Source: CAD feature listing. Evaluate the final solid. Frame: model axes, mm. Face numbers are marked on the shaded views. A direction names the side the tool comes from. Give positions to 0.01 mm unless a question says otherwise; leave off trailing zeros. Order: outer loops, then holes, each group sorted by start corner. A loop starts at its lowest first (then second) coordinate and runs counter-clockwise, first axis right, second up. Notation, with made-up numbers: (31, -13) - (36, -13) arc R15 cw to (36, 15) - close; hole circle Ø6 at (-2.5, 67.25). An arc over 180 degrees is marked (long way). Use CSV: the item, a comma, the result in double quotes.
```python
from build123d import *

# Parameters (mm, degrees)
F1_DEPTH = 49.022
F2_T     = -2.54
F4_W     = 49.022
F4_H     = 1.7985738814
F5_DEPTH = 9.652


with BuildPart() as f1:
    # F0 (on Right) → F1 (new body)
    with BuildSketch(Plane.YZ):
        Polygon((1.5098481488, -2.5384752646), (-15.0794390421, -5.5547094899), (-14.0161000537, -11.4030735567), (1.5098481488, -11.4030735567), (2.9737947043, -19.4547791034), (2.9737947043, -46.7351712286), (-5.6977379136, -46.7351712286), (-5.6886866642, -48.53374511), (16.9632527977, -48.6290739331), (16.9632527977, 26.2930374593), (11.1203547567, 26.2930374593), align=None)
    extrude(amount=-F1_DEPTH)

    # F2
    f2_openings = [f1.faces().sort_by_distance(p)[0] for p in [
        (-24.511, 6.315101, 11.877281),
        (-24.511, -6.784795, -4.046592),
    ]]
    offset(amount=F2_T, openings=f2_openings, kind=Kind.INTERSECTION)

    # F4 (on face) → F5 (join)
    with BuildSketch(Plane.XZ.offset(-2.9737947043)):
        with Locations((-24.511, -47.6344581693)):
            Rectangle(F4_W, F4_H)
    extrude(amount=F5_DEPTH)


with BuildPart() as f8_1:
    # F8: copy of F1
    add(f1.part)


solid = f1.part
```
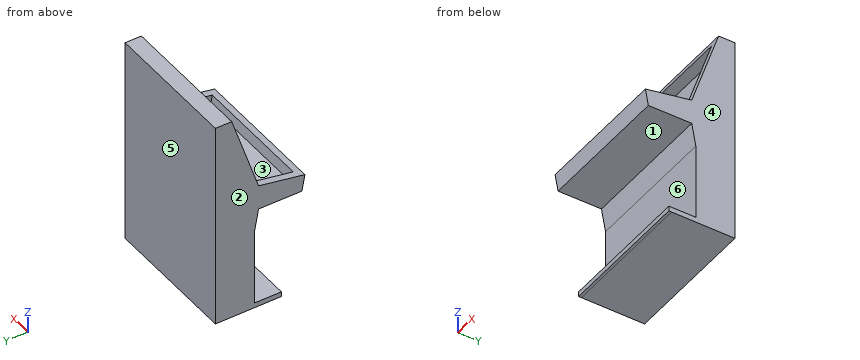
Item 1: Section C-C on y = 8. Return the cut outline in (x, z).
Filled in:
outline,"(-49.02, -48.59) - (0, -48.59) - (0, 16.93) - (-2.54, 16.93) - (-2.54, -46.05) - (-46.48, -46.05) - (-46.48, 16.93) - (-49.02, 16.93) - close"
Item 2: Mould query, pull axis X, two halves, no side actions, for the marked faces 1, 2, 3 and 4. Classes: released by +X, released by -X, zero draft, split by the parting line, or undercut.
Filled in:
face 1,"zero draft"
face 2,"released by -X"
face 3,"undercut"
face 4,"released by +X"
Item 3: Section B-B on x = -39.5. Return the cut outline in (y, z), then the cut area to 3 significant figures.
Filled in:
outline,"(-15.08, -5.55) - (-14.02, -11.4) - (1.51, -11.4) - (2.97, -19.45) - (2.97, -46.74) - (-6.68, -46.74) - (-6.68, -48.53) - (-5.69, -48.53) - (16.96, -48.63) - (16.96, 26.29) - (11.12, 26.29) - (10.27, 23.75) - (14.42, 23.75) - (14.42, -46.08) - (5.51, -46.04) - (5.51, -19.23) - (3.63, -8.86) - (-11.9, -8.86) - (-12.58, -5.1) - close"
area,"390 mm2"
Item 4: Set-up query: the marked faces 5 and 6. Return all of +Z, -Z, +X, -X, +Y, -Y with unobstructed straight access to the full face (end or side cutting, diameter ignored); none if empty.
Filled in:
face 5,"+Z, -Z, +X, -X, +Y"
face 6,"+X, -X, -Y"
Item 5: First-contact query: pin 1 (12 mm diameter, centred on x = -30.5, y = 0, fed in from +Z); pin 2 (0.5 mm diameter, centred on x = -33, y = -6.5, fed in from -Z); pin 3 (22 mm diameter, centred on x = -23.5, z = -32.5, fed in from -Y); pin 4 (1.5 mm diameter, centred on y = 2, z = -25, fed in from -X). Flat tips, straight axial feed; report the tip coordinate or a pass-through.
Filled in:
pin 1,"stops at z = -8.86"
pin 2,"stops at z = -48.53"
pin 3,"stops at y = 2.97"
pin 4,"passes through"
Item 6: Material intervals for line 1 (Z direction, x = -23, y = -4.5); line 2 (X direction, y = 9, z = 5.5); line 3 (Y direction, x = -12, z = -44), sorted ascending. Write a range as from..to.
Filled in:
line 1,"z = -48.54..-46.74, -11.4..-8.86"
line 2,"x = -49.02..-46.48, -2.54..0"
line 3,"y = 2.97..5.51, 14.42..16.96"
Item 7: Section A-A on z = -37. Return the cut outline in (x, y).
Filled in:
outline,"(-49.02, 2.97) - (0, 2.97) - (0, 16.96) - (-49.02, 16.96) - close; hole (-46.48, 5.51) - (-2.54, 5.51) - (-2.54, 14.42) - (-46.48, 14.42) - close"
